Autodesk Inventor part; units mm, degrees
ref_plane "YZ Plane" through (0, 0, 0) normal (1, 0, 0) x (0, 1, 0)
ref_plane "XZ Plane" through (0, 0, 0) normal (0, 1, 0) x (-1, 0, 0)
ref_plane "XY Plane" through (0, 0, 0) normal (0, 0, 1) x (1, 0, 0)
sketch "Sketch_1" plane through (0, 0, 0) normal (0, 0, 1) x (1, 0, 0)
  line L0 (5, 0) -> (-1.5, 0)
  line L1 (-1.5, 0) -> (-1.5, 5)
  line L2 (-1.5, 5) -> (0, 5)
  line L3 (0, 5) -> (0, 3)
  line L4 (0, 3) -> (5, 3)
  line L5 (5, 3) -> (5, 0)
  line L6 (5, 0) -> (-1.5, 0)
revolve "Revolution1" add sketch "Sketch_1" angle 360 about axis through (5, 0, 0) along (1, 0, 0)
sketch "Sketch2" plane through (-1.5, 0, 0) normal (-1, 0, 0) x (0, 0, 1)
  point P0 (0, 0)
hole "Hole1" at (-1.5, 0, 0) direction (1, 0, 0) diameter 2 depth 2 tip angle 120
sketch "Sketch_3" plane through (-1.5, 0, 0) normal (1, 0, 0) x (0, 0, -1)
  line L0 (-1, -0.5774) -> (0, -1.1547)
  line L1 (0, -1.1547) -> (1, -0.5774)
  line L2 (1, -0.5774) -> (1, 0.5774)
  line L3 (1, 0.5774) -> (0, 1.1547)
  line L4 (0, 1.1547) -> (-1, 0.5774)
  line L5 (-1, 0.5774) -> (-1, -0.5774)
extrude "Extrusion1" cut sketch "Sketch_3" along normal blind 2
sketch "Sketch_4" plane through (0, 0, 0) normal (0, 0, 1) x (1, 0, 0)
  line L0 (13, 0) -> (5, 0)
  line L1 (5, 0) -> (5, 2)
  line L2 (5, 2) -> (12.5705, 2)
  line L3 (12.5705, 2) -> (13, 1.5705)
  line L4 (13, 1.5705) -> (13, 0)
  line L5 (13, 0) -> (5, 0)
revolve "Revolution2" add sketch "Sketch_4" angle 360 about axis through (13, 0, 0) along (1, 0, 0)
thread "Thread1"
properties part number "DBGS4-5-8" material "스테인리스스틸"
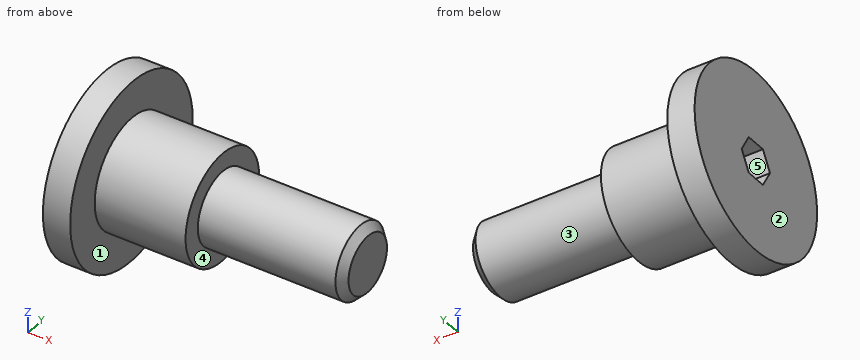
Here's how the part is built. I have some questions about the finished solid (model axes, mm). Face numbers are marked on the shaded views. A direction names the side the tool comes from. Coordinates: 2 decimals unless noted, no trailing zeros. Write each loop counter-clockwise with the first axis right and the second up, starting at its lowest first coordinate (ties: lowest second). Pieces come first, ordered by that corner, then holes. Notation, with made-up numbers: (73, 41.25) -> (132, 41.25) arc R32 ccw to (132, 67.25) -> close; hole circle Ø5 at (3, 42.25). An arc over 180 degrees is marked (long way). Use a Markdown table: item, result. Add a question column.
(1) I'm going to push flat-ended pins straight in: P1, Ø3, axis at x = 9, y = -2.5, coming from the +Z side; P2, Ø4, axis at x = 9.5, z = -2.5, coming from the +Y side; P3, Ø2, axis at x = 3.5, y = -1, coming from the -Z side. Where does each tip first touch, or does it pass through?
(2) If we section it at D-D, the plane x = 10: Write out the boundary of the cut face in (y, z).
(3) If we section it at C-C, the plane y = 2.75: Write out the boundary of the cut face in (x, z), and give its area (3 significant figures).
(4) Please list where these lines run through material, in increasing order: line 1 (X direction, y = 3.5, z = 0.5); line 2 (X direction, y = -1.75, z = -2.25); line 3 (Y direction, x = -1, z = -0.25).
(5) For the marked faces 1 and 2, which set-ups out of +Z, -Z, +X, -X, +Y, -Y let a thin tool reach every point of the face, with its end or its side?
(6) We'd pull the mould along Y, two halves only. Please class the marked faces 3, 4 and 5: +Y half, -Y half, draft (parallel to the pull), parting line (faces both ways), or undercut.
(7) If we section it at B-B, the plane z = -4: Write out the boundary of the cut face in (x, y), and give its area (3 significant figures).
(8) If we section it at A-A, the plane x = -0.5: Write out the boundary of the cut face in (y, z), and give its area (3 significant figures).
Outcome:
| question | item | result |
|---|---|---|
| 1 | P1 | stops at z = 1.73 |
| 1 | P2 | stops at y = 1.94 |
| 1 | P3 | stops at z = -3 |
| 2 | outline | circle Ø4 at (0, 0) |
| 3 | outline | (-1.5, -4.18) -> (0, -4.18) -> (0, -1.2) -> (5, -1.2) -> (5, 1.2) -> (0, 1.2) -> (0, 4.18) -> (-1.5, 4.18) -> close |
| 3 | area | 24.5 mm^2 |
| 4 | line 1 | x = -1.5 to 0 |
| 4 | line 2 | x = -1.5 to 5 |
| 4 | line 3 | y = -4.99 to -1.01, 1.01 to 4.99 |
| 5 | face 1 | +X |
| 5 | face 2 | +Z, -Z, -X, +Y, -Y |
| 6 | face 3 | parting line |
| 6 | face 4 | draft |
| 6 | face 5 | undercut |
| 7 | outline | (-1.5, -3) -> (0, -3) -> (0, 3) -> (-1.5, 3) -> close |
| 7 | area | 9.00 mm^2 |
| 8 | outline | circle Ø10 at (0, 0); hole (-1.15, 0) -> (-0.58, -1) -> (0.58, -1) -> (1.15, 0) -> (0.58, 1) -> (-0.58, 1) -> close |
| 8 | area | 75.1 mm^2 |
